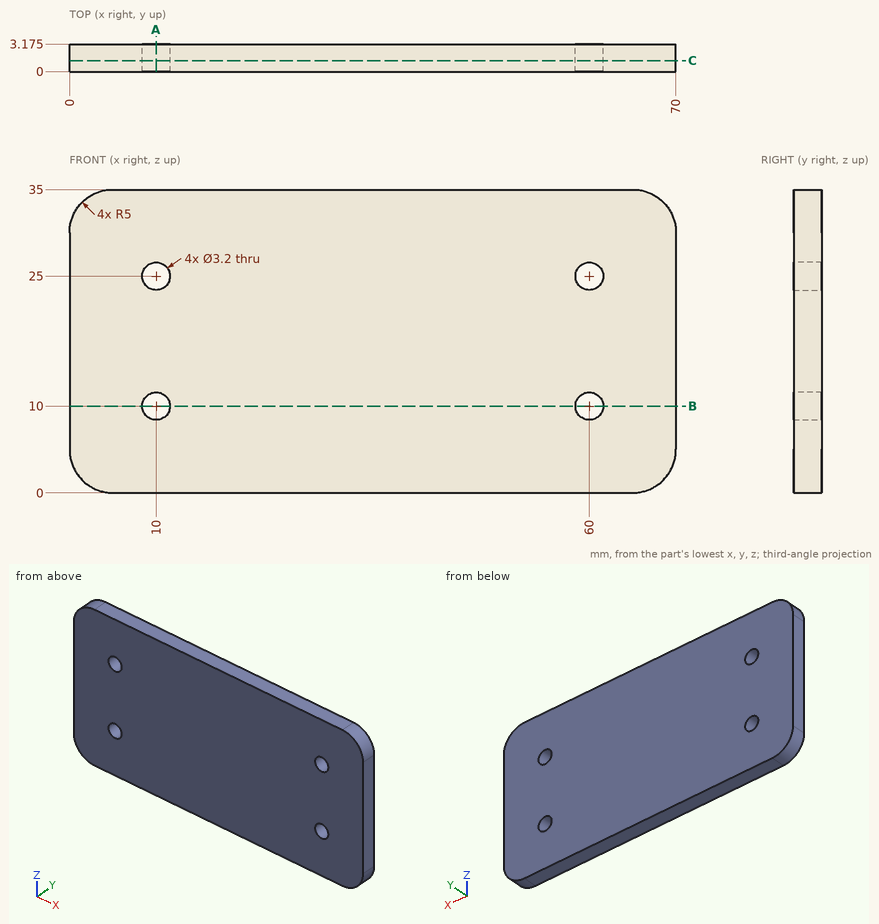
Input: dimensioned drawing with shaded views. Units: mm. Origin: part minimum x, y, z. Round coordinates to 2 decimals unless told otherwise and drop trailing zeros. Order: outer loops, then holes, each group sorted by start corner. A loop starts at its lowest first (then second) coordinate and runs counter-clockwise, first axis right, second up. Notation, with made-up numbers: (87.25, 12.25) -> (110.25, 12.25) arc R33 cw to (110.25, 42.25) -> close; hole circle Ø6 at (27.5, -33.75). An arc over 180 degrees is marked (long way). One line per item, written item: value. Start each with the question number.
Q1. Section query B-B (z = 10). Return the cut outline in (x, y) (3 decimals).
Q2. Pin query (flat end, axial travel): pin 1 (1 mm diameter, centred on x = 26, y = 1, fed in from -Z); pin 2 (2.5 mm diameter, centred on x = 60, z = 25, fed in from +Y). Return the tip coordinate at first contact, or that it passes through.
Q3. Section query C-C (y = 1.25). Return the cut outline in (x, z), plus the area to 3 significant figures.
Q4. Section query A-A (x = 10). Return the cut outline in (y, z) (3 decimals), plus the area to 3 significant figures.
Q5. Material intervals for probe 1 along X at (y, z) = (2.15, 25); probe 2 along Z at (x, y) = (59, 1.45); probe 3 along X at (y, z) = (2.75, 2), sorted ascending.
Findings below:
1. outline: (0, 0) -> (8.4, 0) -> (8.4, 3.175) -> (0, 3.175) -> close; (11.6, 0) -> (58.4, 0) -> (58.4, 3.175) -> (11.6, 3.175) -> close; (61.6, 0) -> (70, 0) -> (70, 3.175) -> (61.6, 3.175) -> close
2. pin 1: z = 0
2. pin 2: through
3. outline: (0, 5) arc R5 ccw to (5, 0) -> (65, 0) arc R5 ccw to (70, 5) -> (70, 30) arc R5 ccw to (65, 35) -> (5, 35) arc R5 ccw to (0, 30) -> close; hole circle Ø3.2 at (10, 10); hole circle Ø3.2 at (10, 25); hole circle Ø3.2 at (60, 10); hole circle Ø3.2 at (60, 25)
3. area: 2,400 mm²
4. outline: (0, 0) -> (3.175, 0) -> (3.175, 8.4) -> (0, 8.4) -> close; (0, 11.6) -> (3.175, 11.6) -> (3.175, 23.4) -> (0, 23.4) -> close; (0, 26.6) -> (3.175, 26.6) -> (3.175, 35) -> (0, 35) -> close
4. area: 90.8 mm²
5. probe 1: 0 to 8.4, 11.6 to 58.4, 61.6 to 70
5. probe 2: 0 to 8.75, 11.25 to 23.75, 26.25 to 35
5. probe 3: 1 to 69
